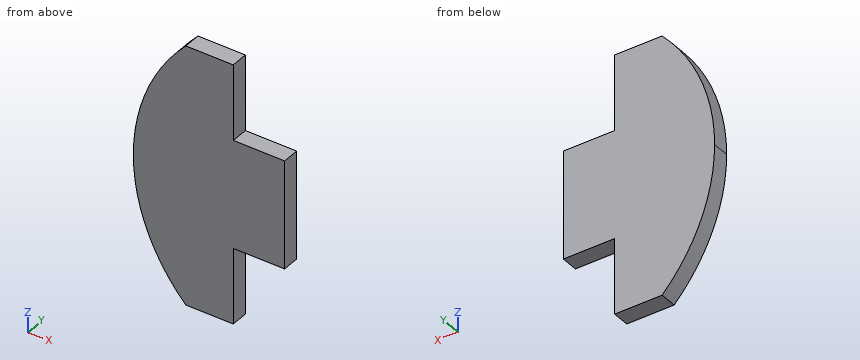
```python
from build123d import *

# Parameters (mm, degrees)
BOSS_EXTRUDE1_DEPTH = 1.6


with BuildPart() as part:
    # Sketch1 → Boss-Extrude1 (new body)
    with BuildSketch(Plane(origin=(0, 0, 0), x_dir=(1, 0, 0), z_dir=(0, 1, 0))):
        with BuildLine():
            Line((-3.25, 0), (-17.25, 0))
            ThreePointArc((-17.25, 0), (-15.989450927, -6.473017771), (-12.392033731, -12))
            Line((-12.392033731, -12), (-8, -12))
            Line((-8, -12), (-8, -5))
            Line((-8, -5), (-3.25, -5))
            Line((-3.25, -5), (-3.25, 0))
        make_face()
        with BuildLine():
            Line((-8, 12), (-12.392033731, 12))
            ThreePointArc((-12.392033731, 12), (-15.989450927, 6.473017771), (-17.25, 0))
            Line((-17.25, 0), (-3.25, 0))
            Line((-3.25, 0), (-3.25, 5))
            Line((-3.25, 5), (-8, 5))
            Line((-8, 5), (-8, 12))
        make_face()
    extrude(amount=BOSS_EXTRUDE1_DEPTH)


solid = part.part
```
Verification items for the finished model (mm, model axes). Coordinates: 2 decimals unless noted, no trailing zeros. Loops run counter-clockwise (first coordinate to the right, second up) from the corner with the lowest first, then second, coordinate; pieces in that order, holes last. Notation, with made-up numbers: (39.25, 32.5) -> (77.25, 32.5) arc R23 cw to (77.25, 50.5) -> close; hole circle Ø8 at (85, -28.5). An arc over 180 degrees is marked (long way). Answer in a Markdown table with one row per item. Add a question column.
1. Material ranges on probe 1 along Z at (x, y) = (-4.75, 1.55); probe 2 along X at (y, z) = (0.3, 6.5); probe 3 along Z at (x, y) = (-13.5, 0.3), recorded low to high. Write a range as [from, to].
2. Section check C-C, the plane z = -4. Enter the section's corners in (x, y).
3. Section check B-B, the plane x = -6. Enter the section's corners in (y, z).
4. Depth check by flat-ended pin: P1, Ø0.8, axis at y = 1, z = -10, coming from the +X side; P2, Ø0.5, axis at x = -6.5, y = 0.5, coming from the +Z side; P3, Ø2, axis at x = -13.5, z = -5, coming from the -Y side; P4, Ø0.8, axis at x = -5.5, y = 1, coming from the -Z side. Enter the tip coordinate at first touch or a pass-through.
5. Section check A-A, the plane y = 1.05. Enter the section's corners in (x, z).
Derived:
| question | item | result |
|---|---|---|
| 1 | probe 1 | z = [-5, 5] |
| 1 | probe 2 | x = [-15.98, -8] |
| 1 | probe 3 | z = [-10.74, 10.74] |
| 2 | outline | (-16.78, 0) -> (-3.25, 0) -> (-3.25, 1.6) -> (-16.78, 1.6) -> close |
| 3 | outline | (0, -5) -> (1.6, -5) -> (1.6, 5) -> (0, 5) -> close |
| 4 | P1 | stops at x = -8 |
| 4 | P2 | stops at z = 5 |
| 4 | P3 | stops at y = 0 |
| 4 | P4 | stops at z = -5 |
| 5 | outline | (-12.39, -12) -> (-8, -12) -> (-8, -5) -> (-3.25, -5) -> (-3.25, 5) -> (-8, 5) -> (-8, 12) -> (-12.39, 12) arc R17.25 ccw to start |
